The listing builds one solid part. Answer for the finished solid, in the listing's coordinates (mm). A direction names the side the tool comes from. Round coordinates to 2 decimals unless told otherwise and drop trailing zeros. Write each loop counter-clockwise with the first axis right and the second up, starting at its lowest first coordinate (ties: lowest second). Pieces come first, ordered by that corner, then holes.
from build123d import *

# Parameters (mm, degrees)
SKETCH1_W           = 128
SKETCH1_H           = 8.4
BOSS_EXTRUDE1_DEPTH = 8
SKETCH2_R           = 1.5
CUT_EXTRUDE1_DEPTH  = 65.634665621
SKETCH3_W           = 108
SKETCH3_H           = 2.8
CUT_EXTRUDE2_DEPTH  = 1
FILLET1_R           = 0.5


with BuildPart() as part:
    # Sketch1 → Boss-Extrude1 (new body)
    with BuildSketch(Plane(origin=(0, 0, 0), x_dir=(1, 0, 0), z_dir=(0, 1, 0))):
        Rectangle(SKETCH1_W, SKETCH1_H)
    extrude(amount=BOSS_EXTRUDE1_DEPTH)

    # Sketch2 → Cut-Extrude1 (cut, through all)
    with BuildSketch(Plane(origin=(0, 8, 0), x_dir=(1, 0, 0), z_dir=(0, 1, 0))):
        with Locations(Location((-60, 0, 0), (0, 0, 270))):
            Circle(SKETCH2_R)
        with Locations(Location((60, 0, 0), (0, 0, 90))):
            Circle(SKETCH2_R)
    extrude(amount=-CUT_EXTRUDE1_DEPTH, mode=Mode.SUBTRACT)

    # Sketch3 → Cut-Extrude2 (cut)
    with BuildSketch(Plane(origin=(0, 8, 0), x_dir=(1, 0, 0), z_dir=(0, 1, 0))):
        Rectangle(SKETCH3_W, SKETCH3_H)
    extrude(amount=-CUT_EXTRUDE2_DEPTH, mode=Mode.SUBTRACT)

    # Fillet1
    fillet1_edges = [part.edges().sort_by_distance(p)[0] for p in [
        (64, 4, 4.2),
        (-64, 4, 4.2),
        (-64, 4, -4.2),
        (64, 4, -4.2),
    ]]
    fillet(fillet1_edges, radius=FILLET1_R)


solid = part.part
1. Section B-B on z = 0 is taken. Determine the outline of the cut face in (x, y).
Geometry says:
outline: (-64, 0) - (-61.5, 0) - (-61.5, 8) - (-64, 8) - close; (-58.5, 0) - (58.5, 0) - (58.5, 8) - (54, 8) - (54, 7) - (-54, 7) - (-54, 8) - (-58.5, 8) - close; (61.5, 0) - (64, 0) - (64, 8) - (61.5, 8) - close
2. Given pin 1 (0.8 mm diameter, centred on x = 24, z = 0, fed in from +Y), flat-ended and moving along its own axis, determine where the tip first touches the part or whether it passes through.
Geometry says:
pin 1: stops at y = 7
3. A tool of negligible diameter and unlimited length cuts with its end or side. For faces 5 (the face through (-1, 4, 4.2)), 6 (the face through (-1, 7, 0)), from which of +Z, -Z, +X, -X, +Y, -Y can it reach the whole face along a straight path? Write none if from no direction.
Geometry says:
face 5: +Z, +X, -X, +Y, -Y
face 6: +Y
4. For a pull along X with two mould halves and no side action, classify faces 1 (the face through (-1, 0, 0)), 2 (the face through (64, 4, 0)), 3 (the face through (58.513, 4.056, 0.195)), 4 (the face through (-64, 4, 0)) as released by +X, released by -X, zero draft, split by the parting line, or undercut.
Geometry says:
face 1: zero draft
face 2: released by +X
face 3: undercut
face 4: released by -X
5. Section A-A on x = 60 is taken. Determine the outline of the cut face in (y, z), plus the area to 3 significant figures.
Geometry says:
outline: (0, -4.2) - (8, -4.2) - (8, -1.5) - (0, -1.5) - close; (0, 1.5) - (8, 1.5) - (8, 4.2) - (0, 4.2) - close
area: 43.2 mm2
6. Section C-C on x = -25.5 is taken. Determine the outline of the cut face in (y, z).
Geometry says:
outline: (0, -4.2) - (8, -4.2) - (8, -1.4) - (7, -1.4) - (7, 1.4) - (8, 1.4) - (8, 4.2) - (0, 4.2) - close
7. Straight lines are drawn through the part: line 1 along X through (y, z) = (5.75, 0); line 2 along Z through (x, y) = (60, 5.75); line 3 along Z through (x, y) = (-30, 7.75). For each, find the intervals that lie inside material, in ascending order.
Geometry says:
line 1: x = -64 to -61.5, -58.5 to 58.5, 61.5 to 64
line 2: z = -4.2 to -1.5, 1.5 to 4.2
line 3: z = -4.2 to -1.4, 1.4 to 4.2
